```python
from build123d import *

# Parameters (mm, degrees)
SKETCH1_R           = 70
SKETCH1_R_2         = 9
BOSS_EXTRUDE1_DEPTH = 2
BOSS_EXTRUDE2_DEPTH = 2
SKETCH5_R           = 1.75
CUT_EXTRUDE4_DEPTH  = 5
CIRPATTERN1_COUNT   = 4
SKETCH3_R           = 1.75
CUT_EXTRUDE2_DEPTH  = 3
CIRPATTERN2_COUNT   = 2
CIRPATTERN2_ANGLE   = 90
SKETCH4_R           = 1.75
CUT_EXTRUDE3_DEPTH  = 3
CIRPATTERN3_COUNT   = 8


with BuildPart() as part:
    # Sketch1 → Boss-Extrude1 (new body)
    with BuildSketch(Plane.XY):
        Circle(SKETCH1_R)
        Circle(SKETCH1_R_2, mode=Mode.SUBTRACT)
    extrude(amount=BOSS_EXTRUDE1_DEPTH)

    # Sketch2 → Boss-Extrude2 (add)
    with BuildSketch(Plane.XY.offset(2)):
        with BuildLine():
            Line((7.47917345, 19.086957969), (15.688781927, 41.642671884))
            ThreePointArc((15.688781927, 41.642671884), (31.466251763, 31.466251763), (41.642671884, 15.688781927))
            Line((41.642671884, 15.688781927), (19.086957969, 7.47917345))
            ThreePointArc((19.086957969, 7.47917345), (14.495689014, 14.495689014), (7.47917345, 19.086957969))
        make_face()
    boss_extrude2 = extrude(amount=BOSS_EXTRUDE2_DEPTH)

    # Sketch5 → Cut-Extrude4 (cut, through all)
    with BuildSketch(Plane.XY.offset(4)):
        with Locations((17.67766953, 24.748737342)):
            Circle(SKETCH5_R)
        with Locations((24.748737342, 17.67766953)):
            Circle(SKETCH5_R)
    cut_extrude4 = extrude(amount=-CUT_EXTRUDE4_DEPTH, mode=Mode.SUBTRACT)

    # CirPattern1: Boss-Extrude2, Cut-Extrude4 ×4 about axis
    cirpattern1_axis = Axis((0, 0, 0), (0, 0, 1))
    for i in range(1, CIRPATTERN1_COUNT):
        add(boss_extrude2.rotate(cirpattern1_axis, i * 360 / CIRPATTERN1_COUNT))
        add(cut_extrude4.rotate(cirpattern1_axis, i * 360 / CIRPATTERN1_COUNT), mode=Mode.SUBTRACT)

    # Sketch3 → Cut-Extrude2 (cut, through all)
    with BuildSketch(Plane.XY.offset(2)):
        with Locations((-12.5, 6)):
            Circle(SKETCH3_R)
        with Locations((12.5, 6)):
            Circle(SKETCH3_R)
        with Locations((12.5, -6)):
            Circle(SKETCH3_R)
        with Locations((-12.5, -6)):
            Circle(SKETCH3_R)
    cut_extrude2 = extrude(amount=-CUT_EXTRUDE2_DEPTH, mode=Mode.SUBTRACT)

    # CirPattern2: Cut-Extrude2 ×2 about axis
    cirpattern2_axis = Axis((0, 0, 0), (0, 0, 1))
    for i in range(1, CIRPATTERN2_COUNT):
        add(cut_extrude2.rotate(cirpattern2_axis, i * CIRPATTERN2_ANGLE / (CIRPATTERN2_COUNT - 1)), mode=Mode.SUBTRACT)

    # Sketch4 → Cut-Extrude3 (cut, through all)
    with BuildSketch(Plane.XY.offset(2)):
        with Locations((0, 65)):
            Circle(SKETCH4_R)
    cut_extrude3 = extrude(amount=-CUT_EXTRUDE3_DEPTH, mode=Mode.SUBTRACT)

    # CirPattern3: Cut-Extrude3 ×8 about axis
    cirpattern3_axis = Axis((0, 0, 0), (0, 0, 1))
    for i in range(1, CIRPATTERN3_COUNT):
        add(cut_extrude3.rotate(cirpattern3_axis, i * 360 / CIRPATTERN3_COUNT), mode=Mode.SUBTRACT)


solid = part.part
```
Input: part model. Units: mm. Frame: model coordinates. A direction names the side the tool comes from. Give positions to 0.01 mm unless a question says otherwise; leave off trailing zeros. Order: outer loops, then holes, each group sorted by start corner. A loop starts at its lowest first (then second) coordinate and runs counter-clockwise, first axis right, second up. Notation, with made-up numbers: M -32.75,80 L 2.25,80 A32 cw 2.25,117 Z; hole C -7,4 d1. An arc over 180 degrees is marked long. Return JSON: item names as keys, results as strings.
1) Section query A-A on z = 3.3. Count the separate pieces of the cut face and the enclosed holes in it, and give its area (3 significant figures).
Taken from the geometry:
{"separate pieces": "4", "enclosed holes": "8", "area": "2,550 mm2"}
2) Access query for faces 4 (the face through (-30.207, 11.527, 2.986)), 5 (the face through (11.527, 30.207, 2.986)), 6 (the face through (-14.41, 14.58, 2.99)), 7 (the face through (30.52, 11.64, 2.99)), 8 (the face through (16.29, 23.68, 2.03)). Directions: +Z, -Z, +X, -X, +Y, -Y. A direction counts if a zero-diameter tool reaches every point of the face in a straight line with its end or side. Return the directions, or none.
Taken from the geometry:
{"face 4": "+Z, -X", "face 5": "+Z, +Y", "face 6": "+Z", "face 7": "+Z, +X", "face 8": "+Z, -Z"}
3) Section query B-B on x = 0. Output: boundary loops of the cut face in (y, z), and give its area (3 significant figures).
Taken from the geometry:
{"outline": "M -70,0 L -66.75,0 L -66.75,2 L -70,2 Z; M -63.25,0 L -9,0 L -9,2 L -63.25,2 Z; M 9,0 L 63.25,0 L 63.25,2 L 9,2 Z; M 66.75,0 L 70,0 L 70,2 L 66.75,2 Z", "area": "230 mm2"}
4) Mould query, pull axis X, two halves, no side actions, for faces 1 (the face through (-31.65, 31.28, 2.99)), 2 (the face through (7.55, 13.31, 1.01)), 3 (the face through (-55.55, -42.594, 0.986)). Classes: released by +X, released by -X, zero draft, split by the parting line, or undercut.
Taken from the geometry:
{"face 1": "released by -X", "face 2": "undercut", "face 3": "split by the parting line"}
5) Section query D-D on y = 12.5. Output: boundary loops of the cut face in (x, z), and give its area (3 significant figures).
Taken from the geometry:
{"outline": "M -68.87,0 L -7.75,0 L -7.75,2 L -16.25,2 L -16.25,4 L -32.88,4 L -32.88,2 L -68.87,2 Z; M -4.25,0 L 4.25,0 L 4.25,2 L -4.25,2 Z; M 7.75,0 L 68.87,0 L 68.87,2 L 32.88,2 L 32.88,4 L 16.25,4 L 16.25,2 L 7.75,2 Z", "area": "328 mm2"}
6) Line query: L1, parallel to Y at x = 0, z = 1.2; L2, parallel to Y at x = -12.5, z = 1.3; L3, parallel to X at y = 18.5, z = 2.5. Output: solid intervals per line, ascending. Write a range as [from, to].
Taken from the geometry:
{"L1": "y = [-70, -66.75], [-63.25, -9], [9, 63.25], [66.75, 70]", "L2": "y = [-68.87, -7.75], [-4.25, 4.25], [7.75, 68.87]", "L3": "x = [-40.47, -26.29], [-23.2, -8.83], [8.83, 23.2], [26.29, 40.47]"}
7) Contact query for flat-ended pins moving along their axis: pin 1 (12 mm diameter, centred on x = 39.5, y = -28, fed in from -Z); pin 2 (3 mm diameter, centred on x = 0, y = 65, fed in from -Z); pin 3 (1.5 mm diameter, centred on x = 31.5, y = 3.5, fed in from +Z); pin 4 (1.5 mm diameter, centred on y = -6.5, z = 1.5, fed in from -X). Output: stop coordinate, or through.
Taken from the geometry:
{"pin 1": "stops at z = 0", "pin 2": "passes through", "pin 3": "stops at z = 2", "pin 4": "stops at x = -69.76"}
8) Section query C-C on y = 65. Output: boundary loops of the cut face in (x, z).
Taken from the geometry:
{"outline": "M -25.98,0 L -1.75,0 L -1.75,2 L -25.98,2 Z; M 1.75,0 L 25.98,0 L 25.98,2 L 1.75,2 Z"}
